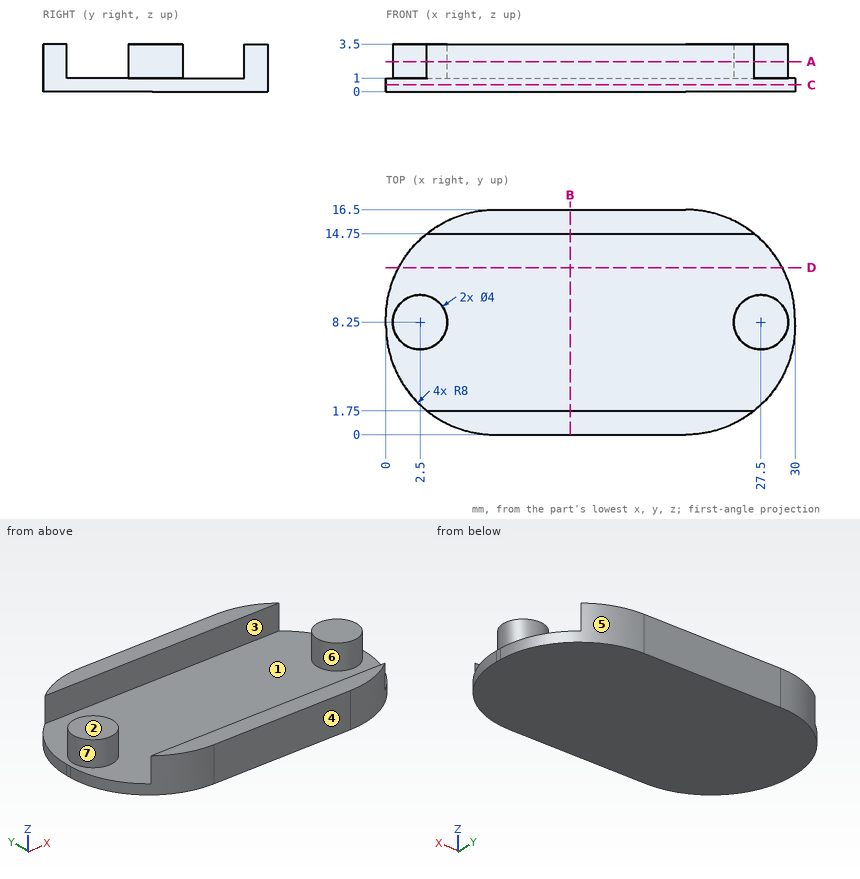
The drawing under review shows one solid part. Ordinate dimensions are in mm from its lowest x, y, z. A direction names the side the tool comes from. Coordinates: 2 decimals unless noted, no trailing zeros. Order: outer loops, then holes, each group sorted by start corner. A loop starts at its lowest first (then second) coordinate and runs counter-clockwise, first axis right, second up. Notation, with made-up numbers: (84.5, 66) -> (90.5, 66) arc R9 cw to (90.5, 71) -> close; hole circle Ø3 at (55, 81). An arc over 180 degrees is marked (long way). Answer in a Markdown table with one row per item. Add a question column.
Item 1: We need section C-C on z = 0.5. Write out the cut boundary in (x, y), plus the area to 3 significant figures.
Item 2: To check wall thickness, follow probe 1 along Y at (x, z) = (14, 1.6); probe 2 along Y at (x, z) = (4, 3.1); probe 3 along Z at (x, y) = (8, 3.25). State the ranges of each line that lie inside material, in increasing order.
Item 3: We need section A-A on z = 2.2. Write out the cut boundary in (x, y).
Item 4: Mouldability with a two-part tool opening along Y and no side actions: class the marked faces 4, 5, 6 and 7 as +Y half, -Y half, draft (parallel to the pull), parting line (faces both ways), or undercut.
Item 5: Clearance check with a flat-ended pin moving along its axis: pin 1 (1.5 mm diameter, centred on x = 18, y = 10, fed in from +Z). State where the tip first meets the part, or that it passes through.
Item 6: We need section D-D on y = 12.25. Write out the cut boundary in (x, z).
Item 7: We need section B-B on x = 13.5. Write out the cut boundary in (y, z).
Item 8: Machinability: for the marked faces 1, 2 and 3, which of the approach directions +Z, -Z, +X, -X, +Y, -Y give a long, thin tool a straight path to every point of the face, cutting with its end or side? Answer none if there is none.
Final values:
| question | item | result |
|---|---|---|
| 1 | outline | (0, 8) arc R8 ccw to (8, 0) -> (22, 0) arc R8 ccw to (30, 8) -> (30, 8.5) arc R8 ccw to (22, 16.5) -> (8, 16.5) arc R8 ccw to (0, 8.5) -> close |
| 1 | area | 440 mm2 |
| 2 | probe 1 | y = 0 to 1.75, 14.75 to 16.5 |
| 2 | probe 2 | y = 1.07 to 1.75, 6.93 to 9.57, 14.75 to 15.43 |
| 2 | probe 3 | z = 0 to 1 |
| 3 | outline | circle Ø4 at (2.5, 8.25); (3.01, 1.75) arc R8 ccw to (8, 0) -> (22, 0) arc R8 ccw to (26.99, 1.75) -> close; (3.01, 14.75) -> (26.99, 14.75) arc R8 ccw to (22, 16.5) -> (8, 16.5) arc R8 ccw to start; circle Ø4 at (27.5, 8.25) |
| 4 | face 4 | -Y half |
| 4 | face 5 | +Y half |
| 4 | face 6 | undercut |
| 4 | face 7 | undercut |
| 5 | pin 1 | stops at z = 1 |
| 6 | outline | (0.93, 0) -> (29.07, 0) -> (29.07, 1) -> (0.93, 1) -> close |
| 7 | outline | (0, 0) -> (16.5, 0) -> (16.5, 3.5) -> (14.75, 3.5) -> (14.75, 1) -> (1.75, 1) -> (1.75, 3.5) -> (0, 3.5) -> close |
| 8 | face 1 | +Z |
| 8 | face 2 | +Z, +X, -X, +Y, -Y |
| 8 | face 3 | +Z, +X, -X |
